Geometry check sheet. Reference: the model listing, model coordinates, mm. Give positions to 0.01 mm unless a question says otherwise; leave off trailing zeros. Order: outer loops, then holes, each group sorted by start corner. A loop starts at its lowest first (then second) coordinate and runs counter-clockwise, first axis right, second up. Notation, with made-up numbers: M 20,22 L 43,22 A22 cw 43,59 Z; hole C -27,45 d2. An arc over 180 degrees is marked long. Answer as CSV lines item,"result". Start each with the question number.
Q1. Section check A-A, the plane x = -25.4. Record the boundary of the cut face in (y, z), then the cut area to 3 significant figures.
Q2. Section check B-B, the plane z = 2.25. Record the boundary of the cut face in (x, y) (1 decimal).
Q3. Section check C-C, the plane x = 12.7. Record the boundary of the cut face in (y, z).
Q4. Section check D-D, the plane y = 10. Record the boundary of the cut face in (x, z).
Q5. Thickness scan on line 1 (Y direction, x = 12.7, z = 2.75); line 2 (Y direction, x = -25.4, z = 3.25); line 3 (X direction, y = -11.5, z = 3.5). Record the ranges inside material, lowest first.
Q6. Go/stop test with flat-tipped pins: pin 1 (3 mm diameter, centred on x = -25.4, y = 0, fed in from -Z); pin 2 (1.5 mm diameter, centred on y = 3.5, z = 1.5, fed in from -X); pin 3 (1 mm diameter, centred on y = -11, z = 2.5, fed in from -X). Record where each tip stops, or that it passes through.
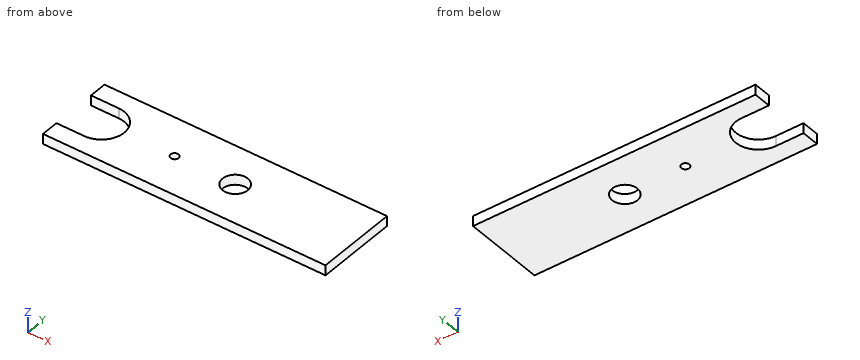
```python
from build123d import *

# Parameters (mm, degrees)
F0_R     = 2.54
F0_R_2   = 7.9375
F1_DEPTH = 6.35


with BuildPart() as f1:
    # F0 (on Top) → F1 (new body)
    with BuildSketch(Plane.XY):
        with BuildLine():
            Line((88.9, -25.4), (88.9, 25.4))
            Line((88.9, 25.4), (-88.9, 25.4))
            Line((-88.9, 25.4), (-88.9, 14.2875))
            Line((-88.9, 14.2875), (-71.4375, 14.2875))
            ThreePointArc((-71.4375, 14.2875), (-57.15, 0), (-71.4375, -14.2875))
            Line((-71.4375, -14.2875), (-88.9, -14.2875))
            Line((-88.9, -14.2875), (-88.9, -25.4))
            Line((-88.9, -25.4), (88.9, -25.4))
        make_face()
        with Locations((-25.4, 0)):
            Circle(F0_R, mode=Mode.SUBTRACT)
        with Locations((12.7, 0)):
            Circle(F0_R_2, mode=Mode.SUBTRACT)
    extrude(amount=F1_DEPTH)


solid = f1.part
```
Answer block:
1,outline,"M -25.4,0 L -2.54,0 L -2.54,6.35 L -25.4,6.35 Z; M 2.54,0 L 25.4,0 L 25.4,6.35 L 2.54,6.35 Z"
1,area,"290 mm2"
2,outline,"M -88.9,-25.4 L 88.9,-25.4 L 88.9,25.4 L -88.9,25.4 L -88.9,14.3 L -71.4,14.3 A14.3 cw -71.4,-14.3 L -88.9,-14.3 Z; hole C -25.4,0 d5.1; hole C 12.7,0 d15.9"
3,outline,"M -25.4,0 L -7.94,0 L -7.94,6.35 L -25.4,6.35 Z; M 7.94,0 L 25.4,0 L 25.4,6.35 L 7.94,6.35 Z"
4,outline,"M -61.23,0 L 88.9,0 L 88.9,6.35 L -61.23,6.35 Z"
5,line 1,"y = -25.4 to -7.94, 7.94 to 25.4"
5,line 2,"y = -25.4 to -2.54, 2.54 to 25.4"
5,line 3,"x = -62.96 to 88.9"
6,pin 1,"passes through"
6,pin 2,"stops at x = -57.8"
6,pin 3,"stops at x = -62.96"
